Work out the finished part from the listing and answer in its coordinate system (mm). A direction names the side the tool comes from. Coordinates: 2 decimals unless noted, no trailing zeros. Order: outer loops, then holes, each group sorted by start corner. A loop starts at its lowest first (then second) coordinate and runs counter-clockwise, first axis right, second up. Notation, with made-up numbers: M 45,79 L 57,79 A11 ccw 57,90 Z; hole C 49,-37 d5. An arc over 180 degrees is marked long. Use a Markdown table: item, result.
from build123d import *

# Parameters (mm, degrees)
F0_W     = 120.5
F0_H     = 172
F1_DEPTH = 11
F2_W     = 97
F2_H     = 120.4
F3_DEPTH = 1
F4_W     = 120.5
F4_H     = 2
F5_DEPTH = 2
F6_W     = 113.7
F6_H     = 9.5
F7_DEPTH = 10.8
F8_W     = 120.5
F8_H     = 12.2
F9_DEPTH = 2


with BuildPart() as f1:
    # F0 (on Front) → F1 (new body)
    with BuildSketch(Plane.XZ):
        with Locations((-66.222898, 72.284041)):
            Rectangle(F0_W, F0_H)
    extrude(amount=F1_DEPTH)

    # F2 (on face) → F3 (cut)
    with BuildSketch(Plane.XZ.offset(11)):
        with Locations((-66.222898, 62.084041)):
            Rectangle(F2_W, F2_H)
    extrude(amount=-F3_DEPTH, mode=Mode.SUBTRACT)

    # F4 (on face) → F5 (join)
    with BuildSketch(Plane.XZ.offset(11)):
        with Locations((-66.222898, 126.284041)):
            Rectangle(F4_W, F4_H)
    extrude(amount=F5_DEPTH)

    # F6 (on face) → F7 (join)
    with BuildSketch(Plane.XY.offset(158.284041)):
        with Locations((-66.222898, -5.5)):
            Rectangle(F6_W, F6_H)
    extrude(amount=F7_DEPTH)

    # F8 (on face) → F9 (join)
    with BuildSketch(Plane.XZ.offset(11)):
        with Locations((-66.222898, 152.184041)):
            Rectangle(F8_W, F8_H)
    extrude(amount=F9_DEPTH)


solid = f1.part
(1) Given P1, Ø5.5, axis at x = -51, z = 136, coming from the -Y side; P2, Ø5, axis at y = -5.5, z = 162.5, coming from the +X side; P3, Ø1.6, axis at x = -58.5, y = -12.5, coming from the -Z side, each flat-ended and moving along its own axis, determine where each tip first touches the part or whether it passes through.
Conclusion:
| item | result |
|---|---|
| P1 | y = -11 |
| P2 | x = -9.37 |
| P3 | z = 125.28 |
(2) A cutting plane is placed at A-A (z = 94.5). Determine the outline of the cut face in (x, y).
Conclusion:
| item | result |
|---|---|
| outline | M -126.47,-11 L -114.72,-11 L -114.72,-10 L -17.72,-10 L -17.72,-11 L -5.97,-11 L -5.97,0 L -126.47,0 Z |
(3) Which of the six approach directions +Z, -Z, +X, -X, +Y, -Y give full straight-line access (tool end or side, diameter ignored) to faces 4 (the flat face through (-67, -11, 137)), 5 (the flat face through (-123.073, -6, 164)), 6 (the flat face through (-67, -10.25, 164)), 7 (the flat face through (-9.373, -6, 164)), 8 (the flat face through (-67, -11, -1))?
Conclusion:
| item | result |
|---|---|
| face 4 | +X, -X, -Y |
| face 5 | +Z, -X, +Y, -Y |
| face 6 | +Z, +X, -X, -Y |
| face 7 | +Z, +X, +Y, -Y |
| face 8 | -Z, +X, -X, -Y |
(4) A cutting plane is placed at C-C (x = -116.5). Determine the outline of the cut face in (y, z).
Conclusion:
| item | result |
|---|---|
| outline | M -13,125.28 L -11,125.28 L -11,-13.72 L 0,-13.72 L 0,158.28 L -0.75,158.28 L -0.75,169.08 L -10.25,169.08 L -10.25,158.28 L -13,158.28 L -13,146.08 L -11,146.08 L -11,127.28 L -13,127.28 Z |
(5) Determine the mould class of faces 1 (the flat face through (-67, -10, 63)), 2 (the flat face through (-67, -5, 169.084)), 3 (the flat face through (-67, -0.75, 164)) for opening direction Z: pulls with the +Z half, pulls with the -Z half, needs draft (parallel to the pull), parting line crosses it, or undercut.
Conclusion:
| item | result |
|---|---|
| face 1 | undercut |
| face 2 | pulls with the +Z half |
| face 3 | needs draft |
(6) A cutting plane is placed at D-D (z = -1). Determine the outline of the cut face in (x, y).
Conclusion:
| item | result |
|---|---|
| outline | M -126.47,-11 L -5.97,-11 L -5.97,0 L -126.47,0 Z |
(7) A cutting plane is placed at B-B (x = -51.5). Determine the outline of the cut face in (y, z).
Conclusion:
| item | result |
|---|---|
| outline | M -13,125.28 L -11,125.28 L -11,122.28 L -10,122.28 L -10,1.88 L -11,1.88 L -11,-13.72 L 0,-13.72 L 0,158.28 L -0.75,158.28 L -0.75,169.08 L -10.25,169.08 L -10.25,158.28 L -13,158.28 L -13,146.08 L -11,146.08 L -11,127.28 L -13,127.28 Z |
(8) Straight lines are drawn through the part: L1, parallel to Z at x = -78.5, y = -11.5; L2, parallel to Z at x = -37.5, y = -10.5; L3, parallel to Y at x = -18, z = -4.5. For each, find the intervals that lie inside material, in ascending order.
Conclusion:
| item | result |
|---|---|
| L1 | 125.28 to 127.28, 146.08 to 158.28 |
| L2 | -13.72 to 1.88, 122.28 to 158.28 |
| L3 | -11 to 0 |
